Source: CAD feature listing. Evaluate the final solid. Frame: model axes, mm. Face numbers are marked on the shaded views. A direction names the side the tool comes from. Coordinates: 2 decimals unless noted, no trailing zeros. Order: outer loops, then holes, each group sorted by start corner. A loop starts at its lowest first (then second) coordinate and runs counter-clockwise, first axis right, second up.
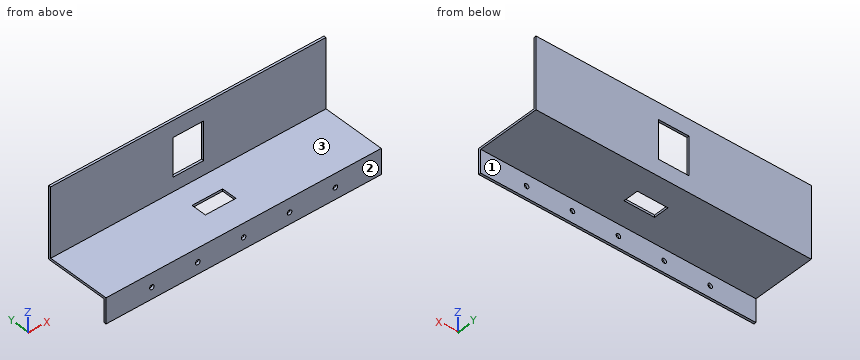
```python
from build123d import *

# Parameters (mm, degrees)
BOSS_EXTRUDE2_DEPTH = 180
SKETCH2_R           = 1.5
CUT_EXTRUDE1_DEPTH  = 10
SKETCH3_W           = 20
SKETCH3_H           = 10
CUT_EXTRUDE2_DEPTH  = 10
SKETCH4_W           = 20
SKETCH4_H           = 25
CUT_EXTRUDE3_DEPTH  = 10


with BuildPart() as part:
    # Sketch1 → Boss-Extrude2 (new body)
    with BuildSketch(Plane(origin=(0, 0, 0), x_dir=(0, 0, -1), z_dir=(1, 0, 0))):
        Polygon((-0.75, 0), (-0.75, 40), (-45.75, 40), (-45.75, 41.5), (0.75, 41.5), (0.75, 0), (15.75, 0), (15.75, -1.5), (-0.75, -1.5), align=None)
    extrude(amount=BOSS_EXTRUDE2_DEPTH)

    # Sketch2 → Cut-Extrude1 (cut)
    with BuildSketch(Plane(origin=(0, 0, 0), x_dir=(1, 0, 0), z_dir=(0, 1, 0))):
        with Locations((120, 8.25)):
            Circle(SKETCH2_R)
        with Locations((90, 8.25)):
            Circle(SKETCH2_R)
        with Locations((150, 8.25)):
            Circle(SKETCH2_R)
        with Locations((60, 8.25)):
            Circle(SKETCH2_R)
        with Locations((30, 8.25)):
            Circle(SKETCH2_R)
    extrude(amount=-CUT_EXTRUDE1_DEPTH, mode=Mode.SUBTRACT)

    # Sketch3 → Cut-Extrude2 (cut)
    with BuildSketch(Plane(origin=(0, 0, -0.75), x_dir=(-1, 0, 0), z_dir=(0, 0, -1))):
        with Locations((-90, 20.75)):
            Rectangle(SKETCH3_W, SKETCH3_H)
    extrude(amount=-CUT_EXTRUDE2_DEPTH, mode=Mode.SUBTRACT)

    # Sketch4 → Cut-Extrude3 (cut)
    with BuildSketch(Plane(origin=(0, 41.5, 0), x_dir=(1, 0, 0), z_dir=(0, 1, 0))):
        with Locations((90, -22.5)):
            Rectangle(SKETCH4_W, SKETCH4_H)
    extrude(amount=-CUT_EXTRUDE3_DEPTH, mode=Mode.SUBTRACT)


solid = part.part
```
Q1. Set-up query: the marked faces 1, 2 and 3. Return all of +Z, -Z, +X, -X, +Y, -Y with unobstructed straight access to the full face (end or side cutting, diameter ignored); none if empty.
Solutions:
face 1: -Z, +X, -X, +Y
face 2: +Z, -Z, +X, -X, -Y
face 3: +Z, +X, -X, -Y
Q2. Section query C-C on x = 138. Output: boundary loops of the cut face in (y, z), plus the area to 4 significant figures.
Solutions:
outline: (-1.5, -15.75) - (0, -15.75) - (0, -0.75) - (41.5, -0.75) - (41.5, 45.75) - (40, 45.75) - (40, 0.75) - (-1.5, 0.75) - close
area: 154.5 mm2
Q3. Section query B-B on y = 24. Output: boundary loops of the cut face in (x, z), plus the area to 3 significant figures.
Solutions:
outline: (0, -0.75) - (80, -0.75) - (80, 0.75) - (0, 0.75) - close; (100, -0.75) - (180, -0.75) - (180, 0.75) - (100, 0.75) - close
area: 240 mm2
Q4. Material intervals for line 1 along X through (y, z) = (-0.7, -8.25); line 2 along Z through (x, y) = (90, -0.7); line 3 along Y through (x, z) = (153, 9), sorted ascending.
Solutions:
line 1: x = 0 to 28.5, 31.5 to 58.5, 61.5 to 88.5, 91.5 to 118.5, 121.5 to 148.5, 151.5 to 180
line 2: z = -15.75 to -9.75, -6.75 to 0.75
line 3: y = 40 to 41.5
Q5. Pin query (flat end, axial travel): P1, Ø8, axis at y = 27, z = -0.5, coming from the -X side; P2, Ø5, axis at x = 25.5, y = 26.5, coming from the -Z side; P3, Ø3, axis at x = 28.5, z = 39.5, coming from the -Y side; P4, Ø5, axis at x = 30, z = -8.25, coming from the +Y side. Return the tip coordinate at first contact, or that it passes through.
Solutions:
P1: stops at x = 0
P2: stops at z = -0.75
P3: stops at y = 40
P4: stops at y = 0
Q6. Section query D-D on z = 7.5. Output: boundary loops of the cut face in (x, y).
Solutions:
outline: (0, 40) - (180, 40) - (180, 41.5) - (0, 41.5) - close
Q7. Section query A-A on z = 17. Output: boundary loops of the cut face in (x, y).
Solutions:
outline: (0, 40) - (80, 40) - (80, 41.5) - (0, 41.5) - close; (100, 40) - (180, 40) - (180, 41.5) - (100, 41.5) - close
